Can you work these out from the model? Positions are in its coordinate system, mm. A direction names the side the tool comes from. Coordinates: 2 decimals unless noted, no trailing zeros. Order: outer loops, then holes, each group sorted by start corner. A loop starts at its lowest first (then second) coordinate and runs counter-clockwise, first axis right, second up. Notation, with made-up numbers: M -18.5,14 L 2.5,14 A21 cw 2.5,19 Z; hole C 15,78.25 d8. An arc over 180 degrees is marked long. Answer as CSV lines item,"result". Start each with the question number.
1. On a 3-axis mill with a long thin cutter (end or side, diameter ignored), from which of +Z, -Z, +X, -X, +Y, -Y can I reach the whole of each face in a straight line? I mean faces 5 (the face through (0, 0, 2)), 6 (the face through (6, -3, 1)), 7 (the face through (0, 3, 37.3)), 8 (the face through (0, 4, 10)). Say none if no direction works.
2. If we section it at D-D (x = -5): List the corners of the cut face in (y, z) for me, plus the area to 3 significant figures.
3. If we section it at A-A (x = 0): List the corners of the cut face in (y, z) for me.
4. If we mould it in two halves opening along Y, with no side actions, what happens to faces 1 (the face through (4.544, 4.002, 1.479)), 2 (the face through (0, -6, 24)), 3 (the face through (1, 4, 5)), 4 (the face through (-0.488, -2.196, 20.39))? For each: released by +Y, released by -Y, zero draft, split by the parting line, or undercut.
5. Will these pins go through, and if not, where does the flat tip stop? pin 1 (5 mm diameter, centred on y = 3, z = 6, fed in from +X); pin 2 (0.6 mm diameter, centred on x = -0.5, z = 1, fed in from +Y); pin 3 (1.3 mm diameter, centred on x = 0, y = -0.5, fed in from +Z).
6. I need wall thicknesses on line 1 along X through (y, z) = (0, 22); line 2 along Z through (x, y) = (-0.5, 4). Which ranges of each line are inside material? Lowest first, please. Write a range as from..to.
7. If we section it at B-B (z = 18): List the corners of the cut face in (x, y) for me, plus the area to 3 significant figures.
```python
from build123d import *

# Parameters (mm, degrees)
F0_R        = 6
F1_DEPTH    = 37.3
F2_W        = 12
F2_H        = 12
F3_DEPTH    = 3
F4_W        = 12
F4_H        = 12.3061701586
F5_DEPTH    = 3.5
F6_W        = 2
F6_H        = 10
F7_DEPTH    = 6
F8_T1_DEPTH = 32.5803989155
F9_W        = 11.8940497642
F9_H        = 34.25
F10_DEPTH   = 6
F11_R       = 2.25
F12_DEPTH   = 34.3
F13_R       = 3


# Not quite as in the source:
# - a fillet or chamfer that OpenCascade refuses, or shapes differently, is made with other operations: its cross-section is extruded or revolved along the edge and cut away or added


with BuildPart() as f1:
    # F0 (on Top) → F1 (new body)
    with BuildSketch(Plane.XY):
        Circle(F0_R)
    extrude(amount=F1_DEPTH)

    # F2 (on face) → F3 (join)
    with BuildSketch(Plane(origin=(0, 0, 0), x_dir=(1, 0, 0), z_dir=(0, 0, -1))):
        Rectangle(F2_W, F2_H)
    extrude(amount=-F3_DEPTH)

    # F4 (on face) → F5 (join)
    with BuildSketch(Plane.XZ.offset(6)):
        with Locations((0, 41.8383553624)):
            Rectangle(F4_W, F4_H)
    extrude(amount=-F5_DEPTH)

    # F6 (on face) → F7 (cut)
    with BuildSketch(Plane(origin=(0, 6, 0), x_dir=(-1, 0, 0), z_dir=(0, 1, 0))):
        with Locations((0, 5)):
            Rectangle(F6_W, F6_H)
    extrude(amount=-F7_DEPTH, mode=Mode.SUBTRACT)

    # F8: fillet of radius 6 on 2 edges, made by hand

    # F8_s2 → F8_t1 (cut)
    with BuildSketch(Plane.XY.offset(-14.7901994578)):
        with BuildLine():
            ThreePointArc((-1, 6), (-4.582575695, 3.9569035631), (-6, 0.0839202169))
            Line((-6, 0.0839202169), (-6, 6))
            Line((-6, 6), (-1, 6))
        make_face()
        with BuildLine():
            ThreePointArc((1, 6), (4.582575695, 3.9569035631), (6, 0.0839202169))
            Line((6, 0.0839202169), (6, 6))
            Line((6, 6), (1, 6))
        make_face()
    extrude(amount=F8_T1_DEPTH, mode=Mode.SUBTRACT)

    # F9 (on face) → F10 (join)
    with BuildSketch(Plane.XZ.offset(6)):
        with Locations((-0.0529751179, 20.125)):
            Rectangle(F9_W, F9_H)
    extrude(amount=-F10_DEPTH)

    # F11 (on face) → F12 (cut)
    with BuildSketch(Plane.XY.offset(37.3)):
        Circle(F11_R)
    extrude(amount=-F12_DEPTH, mode=Mode.SUBTRACT)

    # F13
    f13_edges = [f1.edges().sort_by_distance(p)[0] for p in [
        (6, -4.25, 47.99144),
        (-6, -4.25, 47.99144),
    ]]
    fillet(f13_edges, radius=F13_R)


solid = f1.part
```
Solved:
1,face 5,"+Z, -Z, +Y"
1,face 6,"+Z, -Z, +X, +Y, -Y"
1,face 7,"+Z, +X, -X, +Y"
1,face 8,"-Z, +Y"
2,outline,"M -6,0 L 3.4,0 L 3.4,3 L 3.32,3 L 3.32,37.3 L -2.5,37.3 L -2.5,47.23 L -6,47.23 Z"
2,area,"383 mm²"
3,outline,"M -6,0 L 0,0 L 0,3 L -2.25,3 L -2.25,37.3 L -2.5,37.3 L -2.5,47.99 L -6,47.99 Z; M 2.25,10 L 6,10 L 6,37.3 L 2.25,37.3 Z"
4,face 1,"released by +Y"
4,face 2,"released by -Y"
4,face 3,"zero draft"
4,face 4,"undercut"
5,pin 1,"x = 5.98"
5,pin 2,"y = 0"
5,pin 3,"z = 3"
6,line 1,"-6..-2.25, 2.25..6"
6,line 2,"10..37.3"
7,outline,"M -6,-6 L 5.89,-6 L 5.89,-1.12 A6 ccw long -6,0 Z; hole C 0,0 d4.5"
7,area,"112 mm²"
